Input: dimensioned drawing with shaded views. Units: mm. Origin: part minimum x, y, z. Give positions to 0.01 mm unless a question says otherwise; leave off trailing zeros. Order: outer loops, then holes, each group sorted by start corner. A loop starts at its lowest first (then second) coordinate and runs counter-clockwise, first axis right, second up. Notation, with made-up numbers: M 68.25,7.25 L 74.25,7.25 A30 cw 74.25,29.25 Z; hole C 59.25,31 d8. An arc over 180 degrees is marked long. Answer in a Markdown table with one row per item. Add a question column.
(1) Section query A-A, the plane x = 20. Return loops of the section in (y, z).
(2) Section query C-C, the plane z = 1.45. Count the separate pieces of the cut face and the enclosed holes in it.
(3) Material intervals for line 1 along X through (y, z) = (25, 1.1) (1 decimal); line 2 along X through (y, z) = (6, 0.2) (1 decimal); line 3 along Y through (x, z) = (36, 0.5) (1 decimal), sorted ascending.
(4) Section query D-D, the plane x = 29. Return loops of the section in (y, z) (1 decimal).
(5) Section query B-B, the plane y = 18.5. Return loops of the section in (x, z).
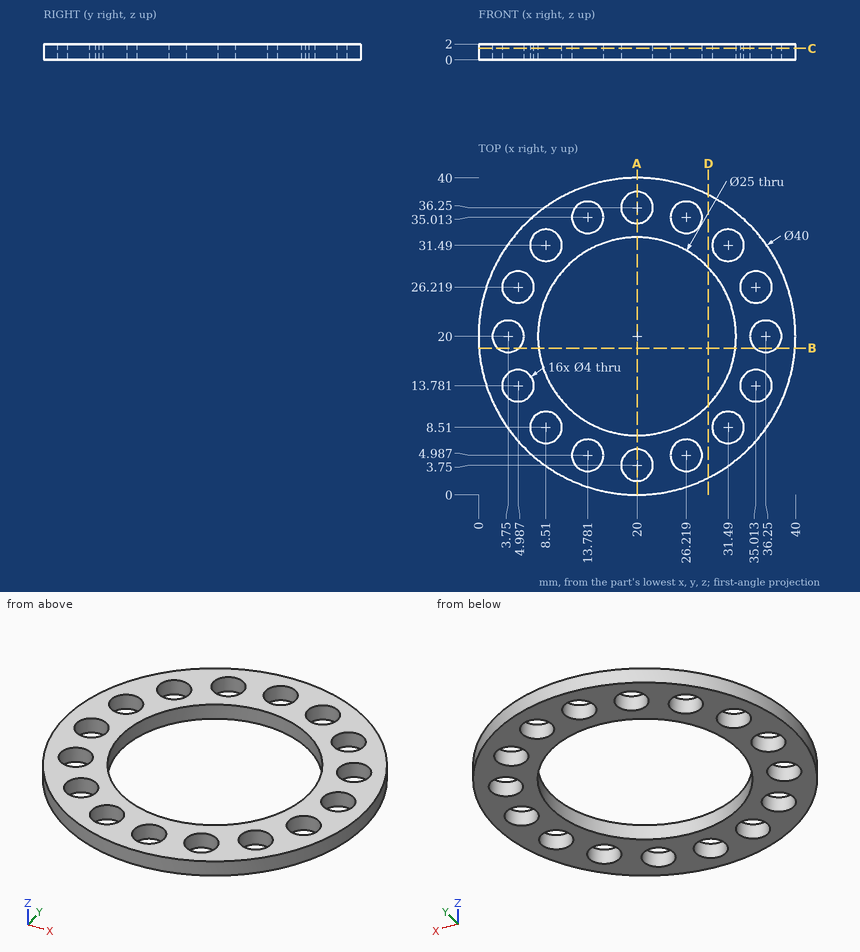
Values follow:
| question | item | result |
|---|---|---|
| 1 | outline | M 0,0 L 1.75,0 L 1.75,2 L 0,2 Z; M 5.75,0 L 7.5,0 L 7.5,2 L 5.75,2 Z; M 32.5,0 L 34.25,0 L 34.25,2 L 32.5,2 Z; M 38.25,0 L 40,0 L 40,2 L 38.25,2 Z |
| 2 | separate pieces | 1 |
| 2 | enclosed holes | 17 |
| 3 | line 1 | x = 0.6 to 3.4, 6.6 to 8.5, 31.5 to 33.4, 36.6 to 39.4 |
| 3 | line 2 | x = 5.7 to 12.1, 15.5 to 24.5, 27.9 to 34.3 |
| 3 | line 3 | y = 8 to 12, 15.5 to 18, 22 to 24.5, 28 to 32 |
| 4 | outline | M 2.1,0 L 11.3,0 L 11.3,2 L 2.1,2 Z; M 28.7,0 L 37.9,0 L 37.9,2 L 28.7,2 Z |
| 5 | outline | M 0.06,0 L 2.43,0 L 2.43,2 L 0.06,2 Z; M 5.07,0 L 7.59,0 L 7.59,2 L 5.07,2 Z; M 32.41,0 L 34.93,0 L 34.93,2 L 32.41,2 Z; M 37.57,0 L 39.94,0 L 39.94,2 L 37.57,2 Z |
